Job drawing, mm, ordinate dimensions from the low corner. One solid piece. A direction names the side the tool comes from. Round coordinates to 2 decimals unless told otherwise and drop trailing zeros. Loops run counter-clockwise (first coordinate to the right, second up) from the corner with the lowest first, then second, coordinate; pieces in that order, holes last.
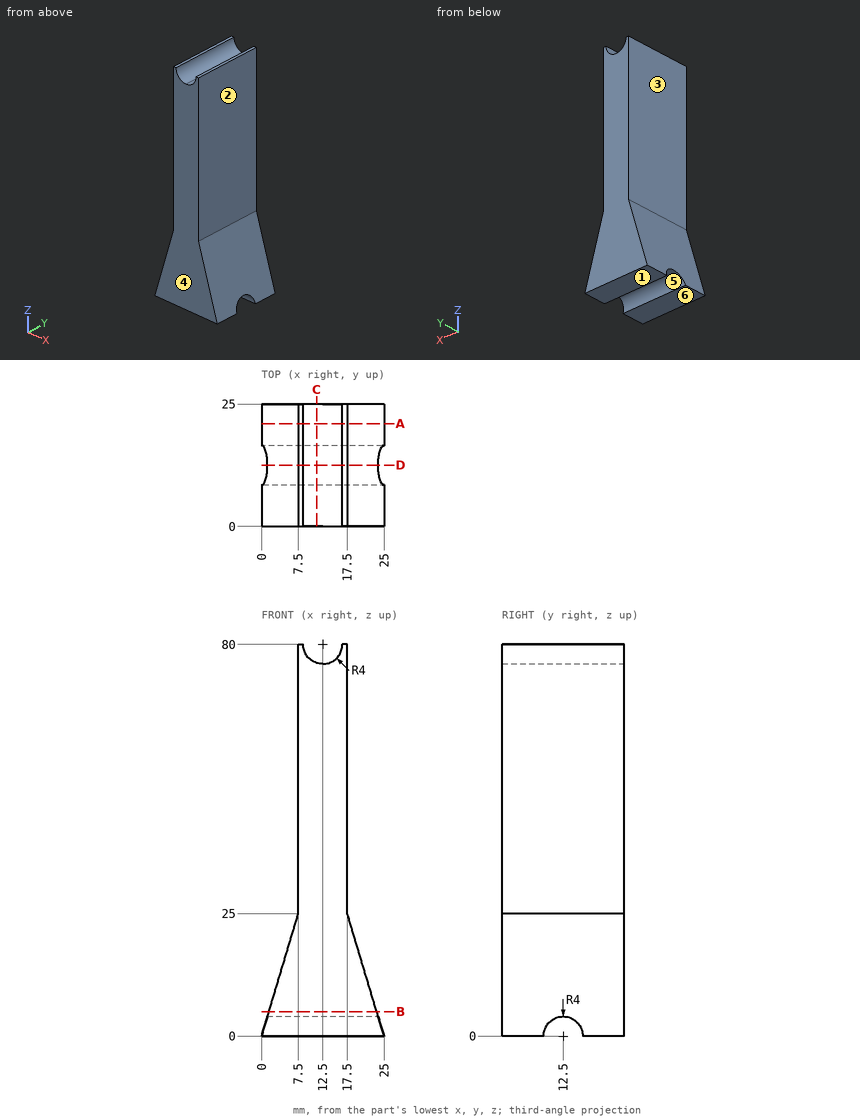
1) Tool access for the marked faces 1, 2 and 3: list every direction of +Z, -Z, +X, -X, +Y, -Y with a clear straight run to the whole face (end or side of a thin tool).
Values:
face 1: -Z, +X, -X, +Y, -Y
face 2: +Z, +X, +Y, -Y
face 3: +Z, -X, +Y, -Y
2) Slice it at A-A, the plane y = 21. Give the cut face in (x, z), then the cut area to 3 significant figures.
Values:
outline: (0, 0) - (25, 0) - (17.5, 25) - (17.5, 80) - (16.5, 80) arc R4 cw to (8.5, 80) - (7.5, 80) - (7.5, 25) - close
area: 962 mm2
3) Mould opens along Y. For the marked faces 4, 5 and 6 say: released by +Y, released by -Y, zero draft, split by the parting line, or undercut.
Values:
face 4: released by -Y
face 5: undercut
face 6: zero draft
4) Drop flat-ended pins along their axis: pin 1 Ø10 at (x, z) = (4, 28.5) entering from -Y; pin 2 Ø1 at (y, z) = (4, 19) entering from -X; pin 3 Ø1 at (x, y) = (15.5, 8) entering from +Z; pin 4 Ø10 at (y, z) = (8.5, 36) entering from +X. Give the stop position or say it passes through.
Values:
pin 1: stops at y = 0
pin 2: stops at x = 5.55
pin 3: stops at z = 78.06
pin 4: stops at x = 17.5
5) Slice it at B-B, the plane z = 5. Give the cut face in (x, y), then the cut area to 3 significant figures.
Values:
outline: (1.5, 0) - (23.5, 0) - (23.5, 25) - (1.5, 25) - close
area: 550 mm2
6) Wall check: line 1 along X through (y, z) = (17, 73.5); line 2 along Y through (x, z) = (13.25, 3); line 3 along Z through (x, y) = (12.5, 7.5). Give the ranges that are in metal, low to high.
Values:
line 1: x = 7.5 to 17.5
line 2: y = 0 to 9.85, 15.15 to 25
line 3: z = 0 to 76
7) Slice it at D-D, the plane y = 12.5. Give the cut face in (x, z).
Values:
outline: (1.2, 4) - (23.8, 4) - (17.5, 25) - (17.5, 80) - (16.5, 80) arc R4 cw to (8.5, 80) - (7.5, 80) - (7.5, 25) - close
8) Slice it at C-C, the plane x = 11.25. Give the cut face in (y, z).
Values:
outline: (0, 0) - (8.5, 0) arc R4 cw to (16.5, 0) - (25, 0) - (25, 76.2) - (0, 76.2) - close
